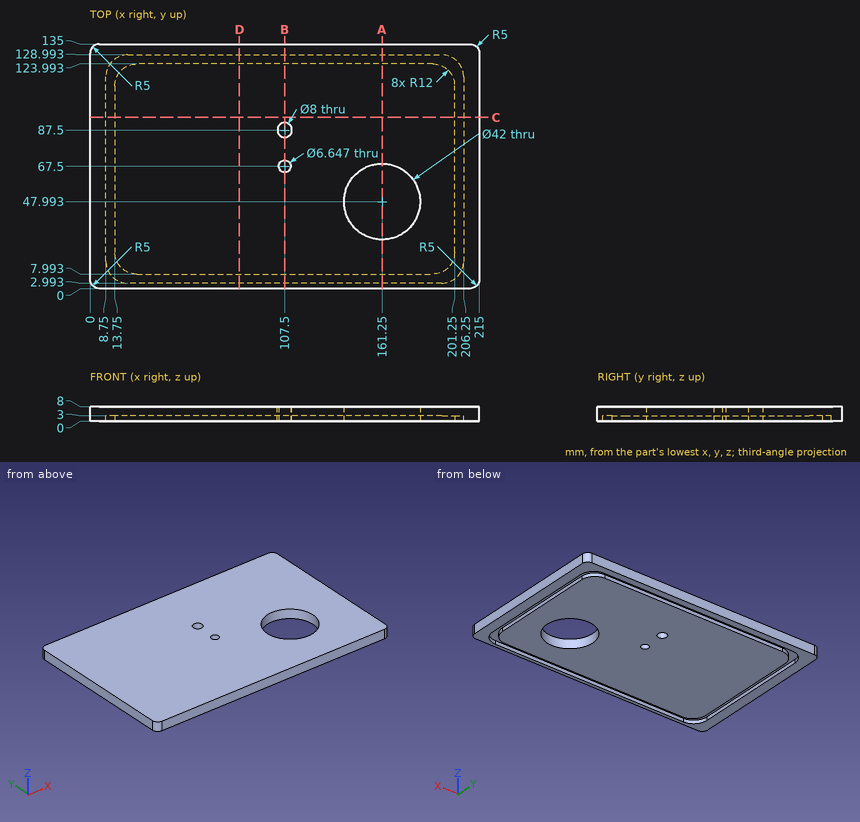
The figure shows three views and two pictorial views of one solid part (mm, origin at its lowest corner). Answer the questions. Give positions to 0.01 mm unless a question says otherwise; leave off trailing zeros. Loops run counter-clockwise (first coordinate to the right, second up) from the corner with the lowest first, then second, coordinate; pieces in that order, holes last. Notation, with made-up numbers: (29.5, 12) -> (86.5, 12) arc R26 ccw to (86.5, 28) -> close; hole circle Ø7 at (-34.75, 29). An arc over 180 degrees is marked (long way). Put each result on its own line as item: value. Start each with the question number.
Item 1: The part is cut by section C-C (y = 94.5). Give the vertices of the cut face in (x, z), then the cut area to 3 significant figures.
Item 2: The part is cut by section B-B (x = 107.5). Give the vertices of the cut face in (y, z).
Item 3: Find the intervals of material crossed by L1, parallel to X at y = 97, z = 2.25; L2, parallel to Y at x = 107.5, z = 6.25; L3, parallel to Y at x = 86.5, z = 2, in increasing order. Write a range as [from, to].
Item 4: The part is cut by section D-D (x = 82.5). Give the vertices of the cut face in (y, z).
Item 5: The part is cut by section A-A (x = 161.25). Give the vertices of the cut face in (y, z), then the cut area to 3 significant figures.
Answers below:
1. outline: (0, 0) -> (8.75, 0) -> (8.75, 3) -> (13.75, 3) -> (13.75, 0) -> (201.25, 0) -> (201.25, 3) -> (206.25, 3) -> (206.25, 0) -> (215, 0) -> (215, 8) -> (0, 8) -> close
1. area: 1,690 mm2
2. outline: (0, 0) -> (2.99, 0) -> (2.99, 3) -> (7.99, 3) -> (7.99, 0) -> (64.18, 0) -> (64.18, 8) -> (0, 8) -> close; (70.82, 0) -> (83.5, 0) -> (83.5, 8) -> (70.82, 8) -> close; (91.5, 0) -> (123.99, 0) -> (123.99, 3) -> (128.99, 3) -> (128.99, 0) -> (135, 0) -> (135, 8) -> (91.5, 8) -> close
3. L1: [0, 8.75], [13.75, 201.25], [206.25, 215]
3. L2: [0, 64.18], [70.82, 83.5], [91.5, 135]
3. L3: [0, 2.99], [7.99, 123.99], [128.99, 135]
4. outline: (0, 0) -> (2.99, 0) -> (2.99, 3) -> (7.99, 3) -> (7.99, 0) -> (123.99, 0) -> (123.99, 3) -> (128.99, 3) -> (128.99, 0) -> (135, 0) -> (135, 8) -> (0, 8) -> close
5. outline: (0, 0) -> (2.99, 0) -> (2.99, 3) -> (7.99, 3) -> (7.99, 0) -> (26.99, 0) -> (26.99, 8) -> (0, 8) -> close; (68.99, 0) -> (123.99, 0) -> (123.99, 3) -> (128.99, 3) -> (128.99, 0) -> (135, 0) -> (135, 8) -> (68.99, 8) -> close
5. area: 714 mm2
